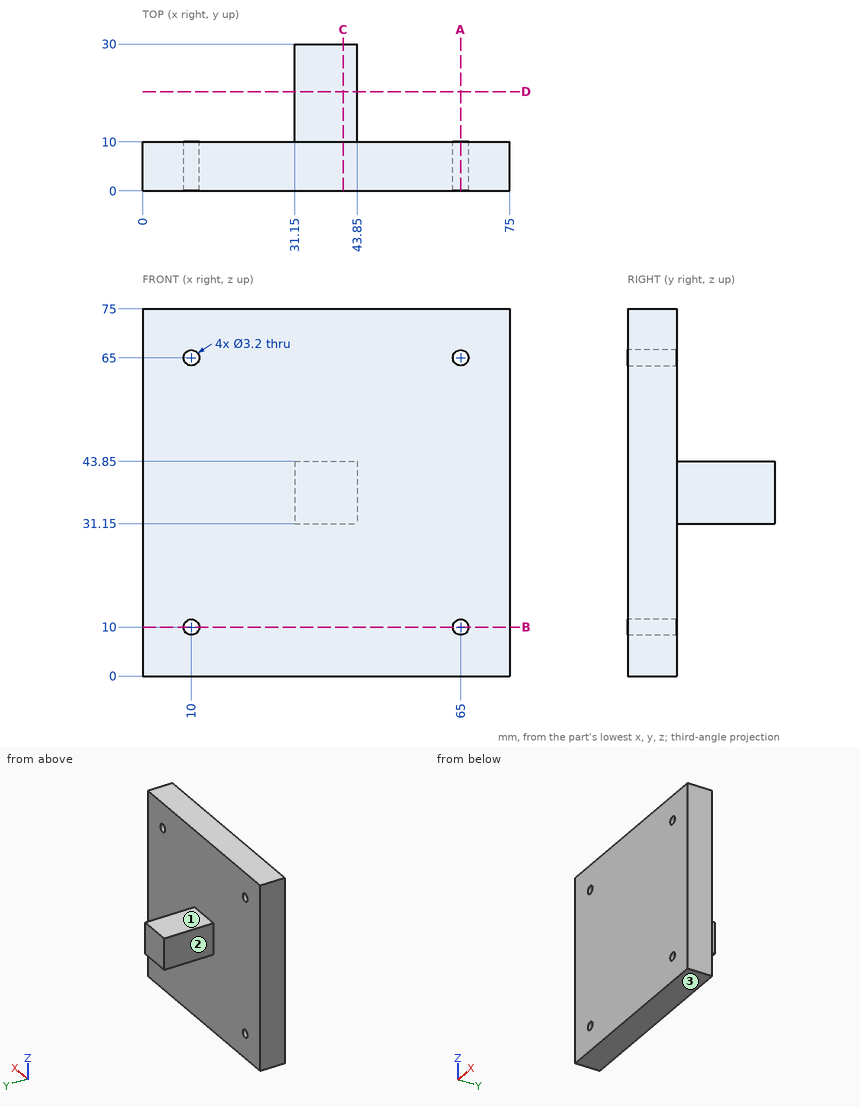
Check sheet for the drawn part. Datum: minimum x, y, z corner. Units: mm. A direction names the side the tool comes from. Coordinates: 2 decimals unless noted, no trailing zeros. Loops run counter-clockwise (first coordinate to the right, second up) from the corner with the lowest first, then second, coordinate; pieces in that order, holes last. Notation, with made-up numbers: (-8, 42.5) -> (10, 42.5) arc R17 ccw to (10, 56.5) -> close; hole circle Ø2 at (9.25, 84). An arc over 180 degrees is marked (long way). Answer as a JSON object with one key per item and string values. Group by question number.
Item 1: Scan lines: probe 1 along X at (y, z) = (3, 10); probe 2 along Y at (x, z) = (7.5, 69.5). Record each from-to range of solid material in increasing order.
Item 2: Tool access check on the marked faces 1, 2 and 3. Record the directions out of +Z, -Z, +X, -X, +Y, -Y that give a thin tool (end or side, any length) a straight path to the whole face; none if there is none.
Item 3: Sectioned sample at A-A on x = 65. Record the boundary of the cut face in (y, z).
Item 4: Sectioned sample at C-C on x = 41. Record the boundary of the cut face in (y, z), plus the area to 3 significant figures.
Item 5: Depth check by flat-ended pin: pin 1 (1.5 mm diameter, centred on x = 25, z = 10.5, fed in from +Y); pin 2 (3.5 mm diameter, centred on x = 65, z = 65, fed in from -Y); pin 3 (14 mm diameter, centred on x = 35.5, y = 22.5, fed in from +Z); pin 4 (6.5 mm diameter, centred on y = 21, z = 35.5, fed in from -X). Enter the tip coordinate at first touch or a pass-through.
Item 6: Sectioned sample at B-B on z = 10. Record the boundary of the cut face in (x, y), plus the area to 3 significant figures.
Item 7: Sectioned sample at D-D on y = 20.25. Record the boundary of the cut face in (x, z), plus the area to 3 significant figures.
Evaluation:
{
 "1": {"probe 1": "x = 0 to 8.4, 11.6 to 63.4, 66.6 to 75", "probe 2": "y = 0 to 10"},
 "2": {"face 1": "+Z, +X, -X, +Y", "face 2": "+Z, -Z, -X, +Y", "face 3": "-Z, +X, -X, +Y, -Y"},
 "3": {"outline": "(0, 0) -> (10, 0) -> (10, 8.4) -> (0, 8.4) -> close; (0, 11.6) -> (10, 11.6) -> (10, 63.4) -> (0, 63.4) -> close; (0, 66.6) -> (10, 66.6) -> (10, 75) -> (0, 75) -> close"},
 "4": {"outline": "(0, 0) -> (10, 0) -> (10, 31.15) -> (30, 31.15) -> (30, 43.85) -> (10, 43.85) -> (10, 75) -> (0, 75) -> close", "area": "1,000 mm²"},
 "5": {"pin 1": "stops at y = 10", "pin 2": "stops at y = 0", "pin 3": "stops at z = 43.85", "pin 4": "stops at x = 31.15"},
 "6": {"outline": "(0, 0) -> (8.4, 0) -> (8.4, 10) -> (0, 10) -> close; (11.6, 0) -> (63.4, 0) -> (63.4, 10) -> (11.6, 10) -> close; (66.6, 0) -> (75, 0) -> (75, 10) -> (66.6, 10) -> close", "area": "686 mm²"},
 "7": {"outline": "(31.15, 31.15) -> (43.85, 31.15) -> (43.85, 43.85) -> (31.15, 43.85) -> close", "area": "161 mm²"}
}
